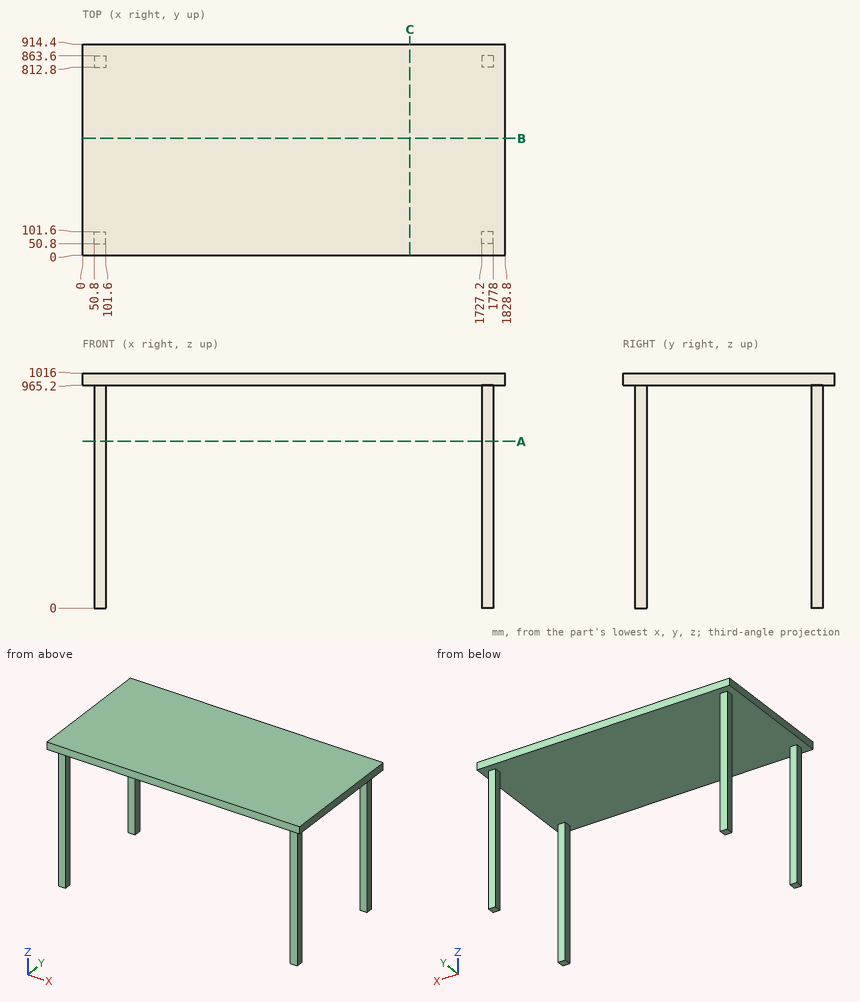
Source: three-view drawing plus pictorial views. Frame: mm from the lowest corner of the part. Round coordinates to 2 decimals unless told otherwise and drop trailing zeros. Loops run counter-clockwise (first coordinate to the right, second up) from the corner with the lowest first, then second, coordinate; pieces in that order, holes last.
1. Section query B-B on y = 506. Output: boundary loops of the cut face in (x, z), and give its area (3 significant figures).
2. Ray query, L1, parallel to X at y = 92, z = 629; L2, parallel to Z at x = 1292, y = 92. Return the intervals inside material, ascending.
3. Contact query for flat-ended pins moving along their axis: pin 1 (15 mm diameter, centred on y = 68.5, z = 446, fed in from +X); pin 2 (15 mm diameter, centred on y = 843.5, z = 551.5, fed in from -X). Output: stop coordinate, or through.
4. Section query C-C on x = 1416.5. Output: boundary loops of the cut face in (y, z).
5. Section query A-A on z = 721.5. Output: boundary loops of the cut face in (x, y).
Answers below:
1. outline: (0, 965.2) - (1828.8, 965.2) - (1828.8, 1016) - (0, 1016) - close
1. area: 92,900 mm2
2. L1: x = 50.8 to 101.6, 1727.2 to 1778
2. L2: z = 965.2 to 1016
3. pin 1: stops at x = 1778
3. pin 2: stops at x = 50.8
4. outline: (0, 965.2) - (914.4, 965.2) - (914.4, 1016) - (0, 1016) - close
5. outline: (50.8, 50.8) - (101.6, 50.8) - (101.6, 101.6) - (50.8, 101.6) - close; (50.8, 812.8) - (101.6, 812.8) - (101.6, 863.6) - (50.8, 863.6) - close; (1727.2, 50.8) - (1778, 50.8) - (1778, 101.6) - (1727.2, 101.6) - close; (1727.2, 812.8) - (1778, 812.8) - (1778, 863.6) - (1727.2, 863.6) - close
